Geometry check sheet. Reference: the model listing, model coordinates, mm. Coordinates: 2 decimals unless noted, no trailing zeros. Write each loop counter-clockwise with the first axis right and the second up, starting at its lowest first coordinate (ties: lowest second). Pieces come first, ordered by that corner, then holes. Notation, with made-up numbers: (-17.75, 13) -> (-4.75, 13) arc R4 cw to (-4.75, 19) -> close; hole circle Ø11 at (-31.5, -3.75). An arc over 180 degrees is marked (long way). Answer in a Markdown table with one row per item. Add a question column.
Q1. Section check A-A, the plane y = 52.5. Count the separate pieces of the cut face and the enclosed holes in it, and give its area (3 significant figures).
Q2. Section check D-D, the plane x = 41. Record the boundary of the cut face in (y, z).
Q3. Thickness scan on line 1 (Z direction, x = 131.5, y = 47.5); line 2 (X direction, y = 42.25, z = -38.42); line 3 (X direction, y = 54, z = -94). Record the ranges inside material, lowest first.
Q4. Section check C-C, the plane z = -29. Record the boundary of the cut face in (x, y).
Q5. Release check for a two-part mould opening along Z. For faces 1 (the face through (18.4, 57, -87.8)), 2 (the face through (148, 30, -99)) record: pulls with the +Z half, pulls with the -Z half, needs draft (parallel to the pull), parting line crosses it, or undercut.
Q6. Gauge pin test, flat ends, axial feed: P1, Ø4, axis at x = 47.5, z = -39.5, coming from the -Y side; P2, Ø3.5, axis at x = 5, z = -95, coming from the -Y side; P3, Ø2, axis at x = 63.96, z = -38.42, coming from the -Y side. Record the tip position at first contact, or that the pin passes through.
```python
from build123d import *

# Parameters (mm, degrees)
SKETCH1_W               = 150
SKETCH1_H               = 100
BOSS_EXTRUDE1_DEPTH     = 60
SHELL1_T                = -3
SKETCH2_W               = 4
SKETCH2_H               = 4
BOSS_EXTRUDE2_DEPTH     = 20
SKETCH3_R               = 0.85
CUT_EXTRUDE1_DEPTH      = 10
SKETCH4_W               = 51
SKETCH4_H               = 28.5
BOSS_EXTRUDE3_DEPTH     = 57
SKETCH5_W               = 49
SKETCH5_H               = 26.5
CUT_EXTRUDE2_DEPTH      = 17.5
SKETCH6_W               = 7.316020892
SKETCH6_H               = 10.063527081
SKETCH6_W_2             = 9.991581276
SKETCH6_H_2             = 9.876768552
CUT_EXTRUDE3_DEPTH      = 1
RIB1_REACH              = 188.304
SKETCH7_WALLS_W         = 497.226705155
SKETCH7_WALLS_H         = 2
SKETCH7_WALLS_W_2       = 2
SKETCH7_WALLS_H_2       = 447.528019614
SKETCH7_WALLS_H_3       = 446.492630332
SKETCH7_WALLS_H_4       = 428.743099781
SKETCH7_WALLS_W_3       = 498.853745456
SKETCH8_W               = 7
SKETCH8_H               = 7
BOSS_EXTRUDE4_DEPTH     = 57
MIRROR2_COPY_1_SKETCH_W = 7
MIRROR2_COPY_1_SKETCH_H = 7
MIRROR2_COPY_1_DEPTH    = 57
SKETCH9_R               = 2
CUT_EXTRUDE4_DEPTH      = 10
MIRROR4_COPY_1_SKETCH_R = 2
MIRROR4_COPY_1_DEPTH    = 10
FILLET1_R               = 5


with BuildPart() as part:
    # Sketch1 → Boss-Extrude1 (new body)
    with BuildSketch(Plane(origin=(0, 0, 0), x_dir=(1, 0, 0), z_dir=(0, 1, 0))):
        with Locations((75, 50)):
            Rectangle(SKETCH1_W, SKETCH1_H)
    extrude(amount=BOSS_EXTRUDE1_DEPTH)

    # Shell1
    shell1_openings = [part.faces().sort_by_distance(p)[0] for p in [
        (75, 0, -50),
    ]]
    offset(amount=SHELL1_T, openings=shell1_openings, kind=Kind.INTERSECTION)

    # Sketch2 → Boss-Extrude2 (add)
    with BuildSketch(Plane.XZ.offset(-57)):
        with Locations((20, -90)):
            Rectangle(SKETCH2_W, SKETCH2_H)
        with Locations((64.26, -90)):
            Rectangle(SKETCH2_W, SKETCH2_H)
        with Locations((20, -38.12)):
            Rectangle(SKETCH2_W, SKETCH2_H)
        with Locations((64.26, -38.12)):
            Rectangle(SKETCH2_W, SKETCH2_H)
    extrude(amount=BOSS_EXTRUDE2_DEPTH)

    # Sketch3 → Cut-Extrude1 (cut)
    with BuildSketch(Plane.XZ.offset(-37)):
        with Locations(Location((20.3, -89.7, 0), (0, 0, 270))):
            Circle(SKETCH3_R)
        with Locations(Location((20.3, -38.42, 0), (0, 0, 270))):
            Circle(SKETCH3_R)
        with Locations(Location((63.96, -38.42, 0), (0, 0, 270))):
            Circle(SKETCH3_R)
        with Locations(Location((63.96, -89.7, 0), (0, 0, 270))):
            Circle(SKETCH3_R)
    extrude(amount=-CUT_EXTRUDE1_DEPTH, mode=Mode.SUBTRACT)

    # Sketch4 → Boss-Extrude3 (add)
    with BuildSketch(Plane.XZ.offset(-57)):
        with Locations((45.5, -20.25)):
            Rectangle(SKETCH4_W, SKETCH4_H)
    extrude(amount=BOSS_EXTRUDE3_DEPTH)

    # Sketch5 → Cut-Extrude2 (cut)
    with BuildSketch(Plane.XZ):
        with Locations((45.5, -20.25)):
            Rectangle(SKETCH5_W, SKETCH5_H)
    extrude(amount=-CUT_EXTRUDE2_DEPTH, mode=Mode.SUBTRACT)

    # Sketch6 → Cut-Extrude3 (cut)
    with BuildSketch(Plane(origin=(71, 0, 0), x_dir=(0, 0, -1), z_dir=(1, 0, 0))):
        with Locations((27.946274495, 5.031763541)):
            Rectangle(SKETCH6_W, SKETCH6_H)
        with Locations((13.255259514, 4.938384276)):
            Rectangle(SKETCH6_W_2, SKETCH6_H_2)
    extrude(amount=-CUT_EXTRUDE3_DEPTH, mode=Mode.SUBTRACT)

    # Sketch7 walls → Rib1 (add, up to next)
    with BuildSketch(Plane(origin=(0, 47, 0), x_dir=(-1, 0, 0), z_dir=(0, -1, 0)), mode=Mode.PRIVATE) as rib1_sk1:
        with Locations((-74.334392604, 80.691896577)):
            Rectangle(SKETCH7_WALLS_W, SKETCH7_WALLS_H)
    rib1_tool1 = extrude(rib1_sk1.sketch, amount=-RIB1_REACH, mode=Mode.PRIVATE) - part.part
    # Sketch7 walls → Rib1 (add, up to next)
    with BuildSketch(Plane(origin=(0, 47, 0), x_dir=(-1, 0, 0), z_dir=(0, -1, 0)), mode=Mode.PRIVATE) as rib1_sk2:
        with Locations((-75.443738264, 51.479127546)):
            Rectangle(SKETCH7_WALLS_W_2, SKETCH7_WALLS_H_2)
    rib1_tool2 = extrude(rib1_sk2.sketch, amount=-RIB1_REACH, mode=Mode.PRIVATE) - part.part
    # Sketch7 walls → Rib1 (add, up to next)
    with BuildSketch(Plane(origin=(0, 47, 0), x_dir=(-1, 0, 0), z_dir=(0, -1, 0)), mode=Mode.PRIVATE) as rib1_sk3:
        with Locations((-118.338437094, 50.961432905)):
            Rectangle(SKETCH7_WALLS_W_2, SKETCH7_WALLS_H_3)
    rib1_tool3 = extrude(rib1_sk3.sketch, amount=-RIB1_REACH, mode=Mode.PRIVATE) - part.part
    # Sketch7 walls → Rib1 (add, up to next)
    with BuildSketch(Plane(origin=(0, 47, 0), x_dir=(-1, 0, 0), z_dir=(0, -1, 0)), mode=Mode.PRIVATE) as rib1_sk4:
        with Locations((-35.211469016, 65.01314459)):
            Rectangle(SKETCH7_WALLS_W_2, SKETCH7_WALLS_H_4)
    rib1_tool4 = extrude(rib1_sk4.sketch, amount=-RIB1_REACH, mode=Mode.PRIVATE) - part.part
    # Sketch7 walls → Rib1 (add, up to next)
    with BuildSketch(Plane(origin=(0, 47, 0), x_dir=(-1, 0, 0), z_dir=(0, -1, 0)), mode=Mode.PRIVATE) as rib1_sk5:
        with Locations((-73.520872454, 57.173768597)):
            Rectangle(SKETCH7_WALLS_W_3, SKETCH7_WALLS_H)
    rib1_tool5 = extrude(rib1_sk5.sketch, amount=-RIB1_REACH, mode=Mode.PRIVATE) - part.part
    add(rib1_tool1.solids().sort_by_distance((74.334392604, 47, -80.691896577))[0])
    add(rib1_tool2.solids().sort_by_distance((75.443738264, 47, -51.479127546))[0])
    add(rib1_tool3.solids().sort_by_distance((118.338437094, 47, -50.961432905))[0])
    add(rib1_tool4.solids().sort_by_distance((35.211469016, 47, -65.01314459))[0])
    add(rib1_tool5.solids().sort_by_distance((73.520872454, 47, -57.173768597))[0])

    # Sketch8 → Boss-Extrude4 (add)
    with BuildSketch(Plane.XZ.offset(-57)):
        with Locations((6.5, -6.5)):
            Rectangle(SKETCH8_W, SKETCH8_H)
    boss_extrude4 = extrude(amount=BOSS_EXTRUDE4_DEPTH)

    # Mirror1: Boss-Extrude4 across plane
    add(boss_extrude4.mirror(Plane.XY.offset(-50)))

    # Mirror2: Boss-Extrude4 across plane
    add(boss_extrude4.mirror(Plane.ZY.offset(-75)))

    # Mirror2 copy 1 sketch → Mirror2 copy 1 (add)
    with BuildSketch(Plane(origin=(150, 57, -100), x_dir=(-1, 0, 0), z_dir=(0, -1, 0))):
        with Locations((6.5, -6.5)):
            Rectangle(MIRROR2_COPY_1_SKETCH_W, MIRROR2_COPY_1_SKETCH_H)
    extrude(amount=MIRROR2_COPY_1_DEPTH)

    # Sketch9 → Cut-Extrude4 (cut)
    with BuildSketch(Plane.XZ):
        with Locations(Location((5, -5, 0), (0, 0, 270))):
            Circle(SKETCH9_R)
    cut_extrude4 = extrude(amount=-CUT_EXTRUDE4_DEPTH, mode=Mode.SUBTRACT)

    # Mirror3: Cut-Extrude4 across plane
    add(cut_extrude4.mirror(Plane.XY.offset(-50)), mode=Mode.SUBTRACT)

    # Mirror4: Cut-Extrude4 across plane
    add(cut_extrude4.mirror(Plane.ZY.offset(-75)), mode=Mode.SUBTRACT)

    # Mirror4 copy 1 sketch → Mirror4 copy 1 (cut)
    with BuildSketch(Plane(origin=(150, 0, -100), x_dir=(-1, 0, 0), z_dir=(0, -1, 0))):
        with Locations(Location((5, -5, 0), (0, 0, 270))):
            Circle(MIRROR4_COPY_1_SKETCH_R)
    extrude(amount=-MIRROR4_COPY_1_DEPTH, mode=Mode.SUBTRACT)

    # Fillet1
    fillet1_edges = [part.edges().sort_by_distance(p)[0] for p in [
        (0, 30, -100),
        (150, 30, -100),
        (150, 30, 0),
        (0, 30, 0),
    ]]
    fillet(fillet1_edges, radius=FILLET1_R)


solid = part.part
```
Calculated:
| question | item | result |
|---|---|---|
| 1 | separate pieces | 5 |
| 1 | enclosed holes | 11 |
| 1 | area | 4,210 mm² |
| 2 | outline | (0, -100) -> (60, -100) -> (60, 0) -> (0, 0) -> (0, -3) -> (57, -3) -> (57, -6) -> (0, -6) -> (0, -7) -> (17.5, -7) -> (17.5, -33.5) -> (0, -33.5) -> (0, -34.5) -> (57, -34.5) -> (57, -56.17) -> (47, -56.17) -> (47, -58.17) -> (57, -58.17) -> (57, -79.69) -> (47, -79.69) -> (47, -81.69) -> (57, -81.69) -> (57, -97) -> (0, -97) -> close |
| 3 | line 1 | z = -100 to -97, -81.69 to -79.69, -58.17 to -56.17, -3 to 0 |
| 3 | line 2 | x = 0 to 3, 18 to 19.45, 21.15 to 22, 62.26 to 63.11, 64.81 to 66.26, 147 to 150 |
| 3 | line 3 | x = 0 to 10, 34.21 to 36.21, 74.44 to 76.44, 117.34 to 119.34, 140 to 150 |
| 4 | outline | (0, 0) -> (3, 0) -> (3, 57) -> (20, 57) -> (20, 0) -> (21, 0) -> (21, 17.5) -> (70, 17.5) -> (70, 10.06) -> (71, 10.06) -> (71, 57) -> (74.44, 57) -> (74.44, 47) -> (76.44, 47) -> (76.44, 57) -> (117.34, 57) -> (117.34, 47) -> (119.34, 47) -> (119.34, 57) -> (147, 57) -> (147, 0) -> (150, 0) -> (150, 60) -> (0, 60) -> close |
| 5 | face 1 | undercut |
| 5 | face 2 | pulls with the -Z half |
| 6 | P1 | stops at y = 57 |
| 6 | P2 | stops at y = 10 |
| 6 | P3 | stops at y = 37 |
